```python
from build123d import *

# Parameters (mm, degrees)
SKETCH1_R               = 55
BOSS_EXTRUDE1_DEPTH     = 6
CUT_EXTRUDE1_DEPTH      = 79.012819459
SKETCH4_R               = 16.25
CUT_EXTRUDE2_DEPTH      = 1.6
CUT_EXTRUDE3_DEPTH      = 78.906097322
CUT_EXTRUDE4_DEPTH      = 78.906097322
CUT_EXTRUDE4_DEPTH_BACK = 78.906097322


with BuildPart() as part:
    # Sketch1 → Boss-Extrude1 (new body)
    with BuildSketch(Plane.XY):
        Circle(SKETCH1_R)
    extrude(amount=BOSS_EXTRUDE1_DEPTH)

    # Sketch3 → Cut-Extrude1 (cut, through all)
    with BuildSketch(Plane.XY.offset(6)):
        with BuildLine():
            ThreePointArc((-15.72828907, 37.971448786), (-14.15882038, 41.760481384), (-17.947852978, 43.329950075))
            ThreePointArc((-17.947852978, 43.329950075), (-33.163308038, 33.163308038), (-43.329950075, 17.947852978))
            ThreePointArc((-43.329950075, 17.947852978), (-41.760481384, 14.15882038), (-37.971448786, 15.72828907))
            ThreePointArc((-37.971448786, 15.72828907), (-29.062088707, 29.062088707), (-15.72828907, 37.971448786))
        make_face()
        with BuildLine():
            ThreePointArc((17.947852978, 43.329950075), (14.15882038, 41.760481384), (15.72828907, 37.971448786))
            ThreePointArc((15.72828907, 37.971448786), (29.062088707, 29.062088707), (37.971448786, 15.72828907))
            ThreePointArc((37.971448786, 15.72828907), (41.760481384, 14.15882038), (43.329950075, 17.947852978))
            ThreePointArc((43.329950075, 17.947852978), (33.163308038, 33.163308038), (17.947852978, 43.329950075))
        make_face()
        with BuildLine():
            ThreePointArc((43.329950075, -17.947852978), (41.760481384, -14.15882038), (37.971448786, -15.72828907))
            ThreePointArc((37.971448786, -15.72828907), (29.062088707, -29.062088707), (15.72828907, -37.971448786))
            ThreePointArc((15.72828907, -37.971448786), (14.15882038, -41.760481384), (17.947852978, -43.329950075))
            ThreePointArc((17.947852978, -43.329950075), (33.163308038, -33.163308038), (43.329950075, -17.947852978))
        make_face()
        with BuildLine():
            ThreePointArc((-17.947852978, -43.329950075), (-14.15882038, -41.760481384), (-15.72828907, -37.971448786))
            ThreePointArc((-15.72828907, -37.971448786), (-29.062088707, -29.062088707), (-37.971448786, -15.72828907))
            ThreePointArc((-37.971448786, -15.72828907), (-41.760481384, -14.15882038), (-43.329950075, -17.947852978))
            ThreePointArc((-43.329950075, -17.947852978), (-33.163308038, -33.163308038), (-17.947852978, -43.329950075))
        make_face()
    extrude(amount=-CUT_EXTRUDE1_DEPTH, mode=Mode.SUBTRACT)

    # Sketch4 → Cut-Extrude2 (cut)
    with BuildSketch(Plane.XY.offset(6)):
        Circle(SKETCH4_R)
    extrude(amount=-CUT_EXTRUDE2_DEPTH, mode=Mode.SUBTRACT)

    # Sketch5 → Cut-Extrude3 (cut, through all)
    with BuildSketch(Plane.XY.offset(4.4)):
        with BuildLine():
            Line((-5.656854249, -7.778174593), (-8.838834765, -10.960155108))
            ThreePointArc((-8.838834765, -10.960155108), (-10.960155108, -10.960155108), (-10.960155108, -8.838834765))
            Line((-10.960155108, -8.838834765), (-7.778174593, -5.656854249))
            ThreePointArc((-7.778174593, -5.656854249), (-5.656854249, -5.656854249), (-5.656854249, -7.778174593))
        make_face()
        with BuildLine():
            Line((-9.5, -1.5), (-11.5, -1.5))
            ThreePointArc((-11.5, -1.5), (-13, 0), (-11.5, 1.5))
            Line((-11.5, 1.5), (-9.5, 1.5))
            ThreePointArc((-9.5, 1.5), (-8, 0), (-9.5, -1.5))
        make_face()
        with BuildLine():
            Line((-7.778174593, 5.656854249), (-10.960155108, 8.838834765))
            ThreePointArc((-10.960155108, 8.838834765), (-10.960155108, 10.960155108), (-8.838834765, 10.960155108))
            Line((-8.838834765, 10.960155108), (-5.656854249, 7.778174593))
            ThreePointArc((-5.656854249, 7.778174593), (-5.656854249, 5.656854249), (-7.778174593, 5.656854249))
        make_face()
        with BuildLine():
            Line((5.656854249, 7.778174593), (8.838834765, 10.960155108))
            ThreePointArc((8.838834765, 10.960155108), (10.960155108, 10.960155108), (10.960155108, 8.838834765))
            Line((10.960155108, 8.838834765), (7.778174593, 5.656854249))
            ThreePointArc((7.778174593, 5.656854249), (5.656854249, 5.656854249), (5.656854249, 7.778174593))
        make_face()
        with BuildLine():
            Line((7.778174593, -5.656854249), (10.960155108, -8.838834765))
            ThreePointArc((10.960155108, -8.838834765), (10.960155108, -10.960155108), (8.838834765, -10.960155108))
            Line((8.838834765, -10.960155108), (5.656854249, -7.778174593))
            ThreePointArc((5.656854249, -7.778174593), (5.656854249, -5.656854249), (7.778174593, -5.656854249))
        make_face()
        with BuildLine():
            Line((9.5, 1.5), (11.5, 1.5))
            ThreePointArc((11.5, 1.5), (13, 0), (11.5, -1.5))
            Line((11.5, -1.5), (9.5, -1.5))
            ThreePointArc((9.5, -1.5), (8, 0), (9.5, 1.5))
        make_face()
    extrude(amount=-CUT_EXTRUDE3_DEPTH, mode=Mode.SUBTRACT)

    # Sketch6 → Cut-Extrude4 (cut, two sides: drawn at the far end of the back side and taken through both)
    with BuildSketch(Plane.XY.offset(4.4).offset(-CUT_EXTRUDE4_DEPTH_BACK)):
        with BuildLine():
            Line((-8.399494937, -32.100505062), (8.399494937, -32.100505062))
            ThreePointArc((8.399494937, -32.100505062), (10.52081528, -31.221825406), (11.399494937, -29.100505062))
            Line((11.399494937, -29.100505062), (11.399494937, -9.899494935))
            Line((11.399494937, -9.899494935), (6.717514421, -5.21751442))
            Line((6.717514421, -5.21751442), (-6.717514421, -5.21751442))
            Line((-6.717514421, -5.21751442), (-11.399494937, -9.899494935))
            Line((-11.399494937, -9.899494935), (-11.399494937, -29.100505062))
            ThreePointArc((-11.399494937, -29.100505062), (-10.52081528, -31.221825406), (-8.399494937, -32.100505062))
        make_face()
        with BuildLine():
            Line((8.399494937, 32.100505063), (-8.399494937, 32.100505063))
            ThreePointArc((-8.399494937, 32.100505063), (-10.52081528, 31.221825407), (-11.399494937, 29.100505063))
            Line((-11.399494937, 29.100505063), (-11.399494937, 9.899494937))
            Line((-11.399494937, 9.899494937), (-6.717514421, 5.217514421))
            Line((-6.717514421, 5.217514421), (6.717514421, 5.217514421))
            Line((6.717514421, 5.217514421), (11.399494937, 9.899494937))
            Line((11.399494937, 9.899494937), (11.399494937, 29.100505063))
            ThreePointArc((11.399494937, 29.100505063), (10.52081528, 31.221825407), (8.399494937, 32.100505063))
        make_face()
    extrude(amount=CUT_EXTRUDE4_DEPTH + CUT_EXTRUDE4_DEPTH_BACK, mode=Mode.SUBTRACT)


solid = part.part
```
CAD build for the part. Positions are in the model's coordinates, mm. A direction names the side the tool comes from. Coordinates: 2 decimals unless noted, no trailing zeros. Order: outer loops, then holes, each group sorted by start corner. A loop starts at its lowest first (then second) coordinate and runs counter-clockwise, first axis right, second up. Notation, with made-up numbers: M 77.5,-40 L 110.5,-40 A24 cw 110.5,-25 Z; hole C -9.5,79.5 d2. An arc over 180 degrees is marked long. Write each question's results on one line, items separated by ' | '. Start each with the question number.
Q1. Cut at C-C (x = 32). List the corners of the cut face in (y, z).
Q2. Pull direction Y, two halves, no side cores. Call faces 3 (the cylindrical face through (16.25, -0.18, 5.21)), 4 (the flat face through (-13, -11, 6)), 5 (the cylindrical face through (-11.923, -53.692, 2.958)): +Y half, -Y half, draft (parallel to the pull), parting line (faces both ways), or undercut.
Q3. Cut at A-A (y = 0). List the corners of the cut face in (x, z).
Q4. Which spindle directions (+Z, -Z, +X, -X, +Y, -Y) get a long thin tool onto all of the face, cutting with end or side? Do faces 1 (the flat face through (0, 0, 4.4)), 2 (the cylindrical face through (32.98, -33.345, 3.042)). Say none if no direction does.
Q5. Cut at D-D (y = 48.5). List the corners of the cut face in (x, z).
Q6. Flat gauge pins, fed straight in: P1, Ø1.8, axis at y = 22, z = 2.5, coming from the +X side; P2, Ø1.3, axis at x = -3, z = 1.5, coming from the +Y side; P3, Ø8, axis at x = 3.5, y = -31.5, coming from the +Z side; P4, Ø1, axis at x = 10.5, z = 1.5, coming from the -Y side. Where does each tip first touch, or does it go through?
Q7. Drill centre lines: probe 1 along Y at (x, z) = (-0.5, 3.8); probe 2 along X at (y, z) = (-16, 1.4); probe 3 along X at (y, z) = (-40.5, 3.55). Where is each one in solid material? Low to high. Write a range as from..to.
Q8. Cut at B-B (x = 0). List the corners of the cut face in (y, z), then the cut area to 3 significant figures.
Found:
1) outline: M -44.73,0 L -34.29,0 L -34.29,6 L -44.73,6 Z; M -25.79,0 L 25.79,0 L 25.79,6 L -25.79,6 Z; M 34.29,0 L 44.73,0 L 44.73,6 L 34.29,6 Z
2) face 3: undercut | face 4: draft | face 5: parting line
3) outline: M -55,0 L -13,0 L -13,4.4 L -16.25,4.4 L -16.25,6 L -55,6 Z; M -8,0 L 8,0 L 8,4.4 L -8,4.4 Z; M 13,0 L 55,0 L 55,6 L 16.25,6 L 16.25,4.4 L 13,4.4 Z
4) face 1: +Z | face 2: +Z, -Z
5) outline: M -25.94,0 L 25.94,0 L 25.94,6 L -25.94,6 Z
6) P1: x = 50.79 | P2: y = 54.95 | P3: z = 6 | P4: y = -54.08
7) probe 1: -55..-32.1, -5.22..5.22, 32.1..55 | probe 2: -52.62..-43.43, -37.86..-11.4, 11.4..37.86, 43.43..52.62 | probe 3: -37.21..-23.65, -13.94..13.94, 23.65..37.21
8) outline: M -55,0 L -32.1,0 L -32.1,6 L -55,6 Z; M -5.22,0 L 5.22,0 L 5.22,4.4 L -5.22,4.4 Z; M 32.1,0 L 55,0 L 55,6 L 32.1,6 Z | area: 321 mm²
